The listing builds one solid part. Answer for the finished solid, in the listing's coordinates (mm). A direction names the side the tool comes from. Round coordinates to 2 decimals unless told otherwise and drop trailing zeros. One line per item, written item: value. Start each with the question number.
1. For a pull along X with two mould halves and no side action, classify faces 1 (the flat face through (0, -65, 16)), 2 (the flat face through (76, 0, 16)), 3 (the cylindrical face through (19.048, -10.435, 24.779)) as released by +X, released by -X, zero draft, split by the parting line, or undercut.
2. A tool of negligible diameter and unlimited length cuts with its end or side. For faces 4 (the cylindrical face through (4.861, -43.733, 24.779)), 5 (the flat face through (153.162, -63, 16)), from which of +Z, -Z, +X, -X, +Y, -Y can it reach the whole face along a straight path? Write none if from no direction.
3. Section A-A, the plane z = 28 is taken. Count the separate pieces of the cut face and the enclosed holes in it, then the cut area to 3 significant figures.
4. A flat-ended cylindrical pin translates along its axis: P1, Ø1.8, axis at x = 58, y = -57, coming from the +Z side. Find the tip coordinate at first contact, or state that the pin passes through.
Autodesk Inventor part; units mm, degrees
ref_plane "YZ Plane" through (0, 0, 0) normal (1, 0, 0) x (0, 1, 0)
ref_plane "XZ Plane" through (0, 0, 0) normal (0, 1, 0) x (-1, 0, 0)
ref_plane "XY Plane" through (0, 0, 0) normal (0, 0, 1) x (1, 0, 0)
sketch "Sketch1" plane through (0, 0, 0) normal (0, 0, 1) x (1, 0, 0)
  line L0 (0, 0) -> (153.162, 0)
  line L1 (153.162, 0) -> (153.162, -127.254)
  line L2 (153.162, -127.254) -> (0, -127.254)
  line L3 (0, -127.254) -> (0, 0)
  dimension "d0" = 153.162
  dimension "d1" = 127.254
extrude "Extrusion1" add sketch "Sketch1" along normal blind 32.004
sketch "Sketch2" plane through (0, 0, 32.004) normal (0, 0, 1) x (1, 0, 0)
  line L0 (0, 0) -> (0, -127.254)
  line L1 (153.162, 0) -> (0, 0)
  circle A0 centre (5.2578, -64.6557) radius 1.8288
  circle A1 centre (5.2578, -57.0865) radius 1.8288
  circle A2 centre (12.827, -57.0865) radius 1.8288
  circle A3 centre (12.827, -64.6557) radius 1.8288
  circle A4 centre (12.827, -49.5173) radius 1.8288
  circle A5 centre (5.2578, -49.5173) radius 1.8288
  circle A6 centre (12.827, -41.9481) radius 1.8288
  circle A7 centre (5.2578, -41.9481) radius 1.8288
  circle A8 centre (20.3962, -64.6557) radius 1.8288
  circle A9 centre (20.3962, -57.0865) radius 1.8288
  circle A10 centre (20.3962, -49.5173) radius 1.8288
  circle A11 centre (5.2578, -34.3789) radius 1.8288
  circle A12 centre (12.827, -34.3789) radius 1.8288
  circle A13 centre (12.827, -26.8097) radius 1.8288
  circle A14 centre (12.827, -19.2405) radius 1.8288
  circle A15 centre (5.26, -19.2405) radius 1.8288
  circle A16 centre (5.2578, -26.8097) radius 1.8288
  circle A17 centre (27.9654, -64.6557) radius 1.8288
  circle A18 centre (27.9654, -57.0865) radius 1.8288
  circle A19 centre (27.9654, -49.5173) radius 1.8288
  circle A20 centre (27.9654, -41.9481) radius 1.8288
  circle A21 centre (27.9654, -34.3789) radius 1.8288
  circle A22 centre (27.9654, -26.8097) radius 1.8288
  circle A23 centre (35.5346, -64.6557) radius 1.8288
  circle A24 centre (35.5346, -57.0865) radius 1.8288
  circle A25 centre (35.5346, -49.5173) radius 1.8288
  circle A26 centre (35.5346, -41.9481) radius 1.8288
  circle A27 centre (35.5346, -34.3789) radius 1.8288
  circle A28 centre (35.5346, -26.8097) radius 1.8288
  circle A29 centre (35.5346, -19.2405) radius 1.8288
  circle A30 centre (27.9654, -19.2405) radius 1.8288
  circle A31 centre (20.3962, -19.2405) radius 1.8288
  circle A32 centre (20.3962, -26.8097) radius 1.8288
  circle A33 centre (20.3962, -34.3789) radius 1.8288
  circle A34 centre (20.3962, -11.6713) radius 1.8288
  circle A35 centre (27.9654, -11.6713) radius 1.8288
  circle A36 centre (35.5346, -11.6713) radius 1.8288
  circle A37 centre (43.1038, -11.6713) radius 1.8288
  circle A38 centre (43.1038, -19.2405) radius 1.8288
  circle A39 centre (43.1038, -26.8097) radius 1.8288
  circle A40 centre (43.1038, -34.3789) radius 1.8288
  circle A41 centre (43.1038, -41.9481) radius 1.8288
  circle A42 centre (43.1038, -49.5173) radius 1.8288
  circle A43 centre (43.1038, -57.0865) radius 1.8288
  circle A44 centre (43.1038, -64.6557) radius 1.8288
  circle A45 centre (50.673, -64.6557) radius 1.8288
  circle A46 centre (58.2422, -64.6557) radius 1.8288
  circle A47 centre (50.673, -57.0865) radius 1.8288
  circle A48 centre (58.2422, -57.0865) radius 1.8288
  circle A49 centre (50.673, -49.5173) radius 1.8288
  circle A50 centre (58.2422, -49.5173) radius 1.8288
  circle A51 centre (58.2422, -41.9481) radius 1.8288
  circle A52 centre (50.673, -41.9481) radius 1.8288
  circle A53 centre (50.673, -34.3789) radius 1.8288
  circle A54 centre (58.2422, -34.3789) radius 1.8288
  circle A55 centre (58.2422, -26.8097) radius 1.8288
  circle A56 centre (50.673, -26.8097) radius 1.8288
  circle A57 centre (50.673, -19.2405) radius 1.8288
  circle A58 centre (58.2422, -19.2405) radius 1.8288
  circle A59 centre (58.2422, -11.6713) radius 1.8288
  circle A60 centre (50.673, -11.6713) radius 1.8288
  circle A61 centre (5.2578, -26.8097) radius 1.8288
  circle A62 centre (5.2578, -11.6713) radius 1.8288
  circle A63 centre (12.827, -11.6713) radius 1.8288
  circle A64 centre (20.3962, -41.9481) radius 1.8288
  circle A65 centre (5.2578, -64.6557) radius 3.175
  circle A66 centre (5.2578, -57.0865) radius 3.175
  circle A67 centre (5.2578, -49.5173) radius 3.175
  circle A68 centre (12.827, -64.6557) radius 3.175
  circle A69 centre (12.827, -57.0865) radius 3.175
  circle A70 centre (12.827, -49.5173) radius 3.175
  circle A71 centre (12.827, -41.9481) radius 3.175
  circle A72 centre (5.2578, -41.9481) radius 3.175
  circle A73 centre (5.2578, -34.3789) radius 3.175
  circle A74 centre (12.827, -34.3789) radius 3.175
  circle A75 centre (20.3962, -64.6557) radius 3.175
  circle A76 centre (20.3962, -57.0865) radius 3.175
  circle A77 centre (20.3962, -49.5173) radius 3.175
  circle A78 centre (20.3962, -41.9481) radius 3.175
  circle A79 centre (20.3962, -34.3789) radius 3.175
  circle A80 centre (20.3962, -26.8097) radius 3.175
  circle A81 centre (12.827, -26.8097) radius 3.175
  circle A82 centre (5.2578, -26.8097) radius 3.175
  circle A83 centre (27.9654, -64.6557) radius 3.175
  circle A84 centre (27.9654, -57.0865) radius 3.175
  circle A85 centre (27.9654, -49.5173) radius 3.175
  circle A86 centre (27.9654, -41.9481) radius 3.175
  circle A87 centre (27.9654, -34.3789) radius 3.175
  circle A88 centre (27.9654, -26.8097) radius 3.175
  circle A89 centre (35.5346, -64.6557) radius 3.175
  circle A90 centre (35.5346, -57.0865) radius 3.175
  circle A91 centre (35.5346, -49.5173) radius 3.175
  circle A92 centre (35.5346, -41.9481) radius 3.175
  circle A93 centre (35.5346, -34.3789) radius 3.175
  circle A94 centre (35.5346, -26.8097) radius 3.175
  circle A95 centre (43.1038, -34.3789) radius 3.175
  circle A96 centre (43.1038, -41.9481) radius 3.175
  circle A97 centre (43.1038, -26.8097) radius 3.175
  circle A98 centre (43.1038, -49.5173) radius 3.175
  circle A99 centre (43.1038, -57.0865) radius 3.175
  circle A100 centre (43.1038, -64.6557) radius 3.175
  circle A101 centre (50.673, -64.6557) radius 3.175
  circle A102 centre (50.673, -57.0865) radius 3.175
  circle A103 centre (50.673, -49.5173) radius 3.175
  circle A104 centre (50.673, -41.9481) radius 3.175
  circle A105 centre (50.673, -34.3789) radius 3.175
  circle A106 centre (58.2422, -64.6557) radius 3.175
  circle A107 centre (58.2422, -57.0865) radius 3.175
  circle A108 centre (58.2422, -49.5173) radius 3.175
  circle A109 centre (58.2422, -41.9481) radius 3.175
  circle A110 centre (58.2422, -34.3789) radius 3.175
  circle A111 centre (58.2422, -26.8097) radius 3.175
  circle A112 centre (50.673, -26.8097) radius 3.175
  circle A113 centre (58.2422, -19.2405) radius 3.175
  circle A114 centre (50.673, -19.2405) radius 3.175
  circle A115 centre (43.1038, -19.2405) radius 3.175
  circle A116 centre (35.5346, -19.2405) radius 3.175
  circle A117 centre (27.9654, -19.2405) radius 3.175
  circle A118 centre (20.3962, -19.2405) radius 3.175
  circle A119 centre (12.827, -19.2405) radius 3.175
  circle A120 centre (5.26, -19.2405) radius 3.175
  circle A121 centre (5.2578, -11.6713) radius 3.175
  circle A122 centre (12.827, -11.6713) radius 3.175
  circle A123 centre (20.3962, -11.6713) radius 3.175
  circle A124 centre (27.9654, -11.6713) radius 3.175
  circle A125 centre (35.5346, -11.6713) radius 3.175
  circle A126 centre (43.1038, -11.6713) radius 3.175
  circle A127 centre (50.673, -11.6713) radius 3.175
  circle A128 centre (58.2422, -11.6713) radius 3.175
  dimension "d4" = 5.2578
  dimension "d5" = 11.6713
  dimension "d6" = 7.5692
  dimension "d7" = 5.26
  dimension "d8" = 7.5692
  dimension "d9" = 5.2578
  dimension "d10" = 7.5692
  dimension "d11" = 7.5692
  dimension "d12" = 5.2578
  dimension "d13" = 7.5692
  dimension "d14" = 7.5692
  dimension "d15" = 7.5692
  dimension "d16" = 7.5692
  dimension "d17" = 7.5692
  dimension "d18" = 7.5692
  dimension "d19" = 7.5692
  dimension "d20" = 7.5692
  dimension "d21" = 7.5692
  dimension "d22" = 7.5692
  dimension "d23" = 3.6576
  dimension "d26" = 3.6576
  dimension "d27" = 3.6576
  dimension "d28" = 3.6576
  dimension "d29" = 3.6576
  dimension "d30" = 3.6576
  dimension "d31" = 3.6576
  dimension "d32" = 3.6576
  dimension "d33" = 3.6576
  dimension "d34" = 3.6576
  dimension "d35" = 3.6576
  dimension "d36" = 3.6576
  dimension "d37" = 3.6576
  dimension "d38" = 3.6576
  dimension "d39" = 3.6576
  dimension "d40" = 3.6576
  dimension "d41" = 3.6576
  dimension "d42" = 3.6576
  dimension "d43" = 3.6576
  dimension "d44" = 3.6576
  dimension "d45" = 3.6576
  dimension "d46" = 3.6576
  dimension "d47" = 3.6576
  dimension "d48" = 3.6576
  dimension "d49" = 3.6576
  dimension "d50" = 3.6576
  dimension "d51" = 3.6576
  dimension "d52" = 3.6576
  dimension "d53" = 3.6576
  dimension "d54" = 3.6576
  dimension "d55" = 3.6576
  dimension "d56" = 3.6576
  dimension "d57" = 3.6576
  dimension "d58" = 3.6576
  dimension "d59" = 3.6576
  dimension "d60" = 3.6576
  dimension "d61" = 3.6576
  dimension "d62" = 3.6576
  dimension "d63" = 3.6576
  dimension "d64" = 3.6576
  dimension "d65" = 3.6576
  dimension "d66" = 3.6576
  dimension "d67" = 3.6576
  dimension "d68" = 3.6576
  dimension "d69" = 3.6576
extrude "Extrusion2" cut sketch "Sketch2" against normal blind 14.6558 contours A0
extrude "Extrusion3" cut sketch "Sketch2" against normal blind 14.6558 contours A0 | A1 | A2 | A3 | A4 | A5 | A6 | A7 | A8 | A9 | A10 | A11 | A12 | A13 | A14 | A15 | A16 | A17 | A18 | A19 | A20 | A21 | A22 | A23 | A24 | A25 | A26 | A27 | A28 | A29 | A30 | A31 | A32 | A33 | A34 | A35 | A36 | A37 | A38 | A39 | A40 | A41 | A42 | A43 | A44 | A45 | A46 | A47 | A48 | A49 | A50 | A51 | A52 | A53 | A54 | A55 | A56 | A57 | A58 | A59 | A60 | A62 | A63 | A64
sketch "Sketch3" plane through (12.827, -49.5173, 17.3482) normal (0, 0, 1) x (1, 0, 0)
  circle A0 centre (-6.5853, 36.1219) radius 5.8342
  circle A1 centre (-7.5692, 37.846) radius 1.8288
  circle A2 centre (-7.5692, 37.846) radius 3.175
  point P0 (-12.827, 49.5173)
  dimension "d92" = 6.35
properties part number "thermocylcer block"
Answer list:
1. face 1: released by -X
1. face 2: zero draft
1. face 3: undercut
2. face 4: +Z
2. face 5: +Z, -Z, +X, +Y, -Y
3. separate pieces: 1
3. enclosed holes: 64
3. area: 18,800 mm²
4. P1: stops at z = 17.35
